Build history of the part. All positions in model axes, mm. Round coordinates to 2 decimals unless told otherwise and drop trailing zeros. Write each loop counter-clockwise with the first axis right and the second up, starting at its lowest first coordinate (ties: lowest second). Pieces come first, ordered by that corner, then holes. Notation, with made-up numbers: (-16, 84.5) -> (-9, 84.5) arc R26 ccw to (-9, 98.5) -> close; hole circle Ø9 at (10.5, -33.75). An arc over 180 degrees is marked (long way). One line per question, with ' | ' between items.
Autodesk Fusion 360 part; units mm, degrees
sketch "Sketch2" plane through (0, 0, 0) normal (0, 1, 0) x (1, 0, 0)
  circle A0 centre (0, 0) radius 80
  circle A1 centre (0, -65) radius 4
  circle A2 centre (-56.2917, 32.5) radius 4
  circle A3 centre (56.2917, 32.5) radius 4
  circle A4 centre (0, 0) radius 23
  dimension "d29" = 160
  dimension "d30" = 8
  dimension "d31" = 8
  dimension "d32" = 8
  dimension "d33" = 120
  dimension "d34" = 120
  dimension "d35" = 65
  dimension "d36" = 65
  dimension "d37" = 65
  dimension "d38" = 46
sketch "Sketch3" plane through (0, 0, 0) normal (0, 1, 0) x (1, 0, 0)
  circle A0 centre (0, -82) radius 3
  circle A1 centre (0, -65) radius 4
  circle A2 centre (37.7308, -33.7512) radius 3
  circle A3 centre (-45.463, -21.7852) radius 3
  circle A4 centre (-5.4604, -38.8527) radius 43.4915 construction
  line L0 (0, 0) -> (0, -106.7199)
  line L1 (0, 0) -> (-5.4604, -38.8527) construction
  circle A5 centre (-5.4604, -38.8527) radius 52.5
  line L2 (-44.0663, -23.3245) -> (-50.9, -23.3245)
  line L3 (-47.433, -26.5975) -> (-47.433, -19.6919)
  line L4 (32.8029, -32.5277) -> (40.5, -32.5277)
  line L5 (36.1117, -35.7471) -> (36.1117, -28.3628)
  point P0 (-47.433, -23.3245)
  point P1 (36.1117, -32.5277)
  dimension "d40" = 6
  dimension "d41" = 17
  dimension "d42" = 6
  dimension "d43" = 61.25
  dimension "d44" = 6
  dimension "d45" = 84.05
  dimension "d46" = 75.45
  dimension "d47" = 8
  dimension "d48" = 105
extrude "Extrude1" add sketch "Sketch3" sketch "Sketch2" along normal blind 10 of sketch 2
extrude "Extrude2" cut sketch "Sketch3" along normal blind 10 contours A0 L0 | A0 L0
extrude "Extrude3" cut sketch "Sketch2" along normal blind 10 contours A4
extrude "Extrude4" cut sketch "Sketch3" along normal blind 10 contours A3 L2 L3 | A3 L2 L3
extrude "Extrude5" cut sketch "Sketch3" along normal blind 10 contours A2 L4 | A2 L4 L5 | A2 L4 L5
sketch "Sketch4" plane through (0, 0, 0) normal (0, -1, 0) x (1, 0, 0)
  circle A0 centre (37.7308, 33.7512) radius 3
  circle A1 centre (-45.463, 21.7852) radius 3
  circle A2 centre (0, 65) radius 4
  circle A3 centre (0, 0) radius 23
  circle A4 centre (56.2917, -32.5) radius 4
  circle A5 centre (-56.2917, -32.5) radius 4
  arc A6 (35.5015, 71.6913) -> (-53.887, 59.1286) centre (-5.4604, 38.8527) ccw
  arc A7 (-53.887, 59.1286) -> (35.5015, 71.6913) centre (0, 0) ccw
  circle A8 centre (0, 82) radius 3
  circle A9 centre (0, 0) radius 23
  circle A10 centre (37.7308, 33.7512) radius 3
  circle A11 centre (0, 65) radius 4
  circle A12 centre (0, 82) radius 3
  circle A13 centre (-45.463, 21.7852) radius 3
  circle A14 centre (-56.2917, -32.5) radius 4
  circle A15 centre (56.2917, -32.5) radius 4
  line L0 (0, 83.5) -> (0, 80)
  line L1 (-1.6, 82) -> (1.6, 82)
  line L2 (0, 67.3) -> (0, 62.5)
  line L3 (-3, 65) -> (3.4, 65)
  line L4 (35.496, 33.7512) -> (39.8, 33.7512)
  line L5 (37.7308, 36.0039) -> (37.7308, 31.5)
  line L6 (-45.463, 24.0048) -> (-45.463, 19.2402)
  line L7 (-47.6513, 21.7852) -> (-43.1669, 21.7852)
  line L8 (-56.2917, -29.4965) -> (-56.2917, -35.5)
  line L9 (-59, -32.5) -> (-53.5, -32.5)
  line L10 (56.2917, -29.0015) -> (56.2917, -36)
  line L11 (53.1873, -32.5) -> (59.5, -32.5)
  line L12 (0, 10) -> (0, -9.5078)
  line L13 (-10, 0) -> (10, 0)
  dimension "d59" = 46
  dimension "d60" = 6
  dimension "d61" = 8
  dimension "d62" = 6
  dimension "d63" = 6
  dimension "d64" = 8
  dimension "d65" = 8
(1) Slice it at B-B (x = 0). Write the cut outline in (y, z).
Calculated:
outline: (0, -80) -> (10, -80) -> (10, -23) -> (0, -23) -> close; (0, 23) -> (10, 23) -> (10, 61) -> (0, 61) -> close; (0, 69) -> (10, 69) -> (10, 79) -> (0, 79) -> close; (0, 85) -> (10, 85) -> (10, 91.07) -> (0, 91.07) -> close
(2) Mould opens along X. For faces 1 (the cylindrical face through (8.308, 4.93, -79.567)), 2 (the cylindrical face through (-0.867, 4.93, 61.095)), 3 (the cylindrical face through (-42.602, 4.93, 22.686)), 4 (the flat face through (-19, 10, -15)) say: pulls with the +X half, pulls with the -X half, needs draft (parallel to the pull), parting line crosses it, or undercut.
Calculated:
face 1: parting line crosses it | face 2: undercut | face 3: undercut | face 4: needs draft
(3) Wall check: line 1 (Z direction, x = 0, y = 3.75); line 2 (X direction, y = 3.25, z = 0); line 3 (Z direction, x = 3.5, y = 7.75). Give the ranges that are in metal, low to high. Write a range as from..to.
Calculated:
line 1: -80..-23, 23..61, 69..79, 85..91.07 | line 2: -80..-23, 23..80 | line 3: -79.92..-22.73, 22.73..63.06, 66.94..90.58
(4) Drop flat-ended pins along their axis: pin 1 (1.5 mm diameter, centred on y = 6, z = 30, fed in from -X); pin 2 (6 mm diameter, centred on x = -51, y = 1.5, fed in from -Z); pin 3 (6 mm diameter, centred on x = 25.5, y = 6.5, fed in from -Z). Give the stop position or say it passes through.
Calculated:
pin 1: x = -74.46 | pin 2: z = -64 | pin 3: z = -76.77
(5) Slice it at D-D (z = 82). Write the cut outline in (x, y).
Calculated:
outline: (-35.37, 0) -> (-3, 0) -> (-3, 10) -> (-35.37, 10) -> close; (3, 0) -> (24.45, 0) -> (24.45, 10) -> (3, 10) -> close
(6) Slice it at C-C (y = 3.75). Write the cut outline in (x, z).
Calculated:
outline: (-53.89, 59.13) arc R80 ccw (long way) to (35.5, 71.69) arc R52.5 ccw to start; hole circle Ø8 at (-56.29, -32.5); hole circle Ø6 at (-45.46, 21.79); hole circle Ø46 at (0, 0); hole circle Ø8 at (0, 65); hole circle Ø6 at (0, 82); hole circle Ø6 at (37.73, 33.75); hole circle Ø8 at (56.29, -32.5)
(7) Slice it at A-A (z = 0). Write the cut outline in (x, y).
Calculated:
outline: (-80, 0) -> (-23, 0) -> (-23, 10) -> (-80, 10) -> close; (23, 0) -> (80, 0) -> (80, 10) -> (23, 10) -> close
